Can you work these out from the model? Positions are in its coordinate system, mm. Give positions to 0.01 mm unless a question says otherwise; leave off trailing zeros. Loops run counter-clockwise (first coordinate to the right, second up) from the corner with the lowest first, then second, coordinate; pieces in that order, holes last. Notation, with made-up numbers: (-28, 9.25) -> (28, 9.25) arc R23 ccw to (28, 43.25) -> close; hole circle Ø8 at (32.25, 65.25). An arc over 180 degrees is marked (long way). Return JSON: item names as keys, results as strings. Group by question number.
Q1. Suppose I cut it at A-A, the plane y = 1.5. Count the separate pieces of the cut face and the enclosed holes in it, and give its area (3 significant figures).
Q2. Will these pins go through, and if not, where does the flat tip stop? pin 1 (5 mm diameter, centred on y = 42, z = 17.5, fed in from +X); pin 2 (2 mm diameter, centred on x = -9, z = 16, fed in from +Y); pin 3 (1.5 mm diameter, centred on y = 15.5, z = 18, fed in from +X).
Q3. Suppose I cut it at B-B, the plane x = 0. Please give me the cut outline in (y, z), and give its area (3 significant figures).
Q4. Suppose I cut it at D-D, the plane x = -24. Please give me the cut outline in (y, z).
Q5. I need wall thicknesses on line 1 along Y through (x, z) = (25, 14); line 2 along X through (y, z) = (27, -2.5); line 3 along Z through (x, y) = (5.5, 51). Which ranges of each line are inside material? Lowest first, please. Write a range as [from, to].
Q6. Suppose I cut it at C-C, the plane z = 18.5. Please give me the cut outline in (x, y), and give its area (3 significant figures).
Q7. Thinking about a two-plate mould opening in X: for faces 1 (the flat face through (-14.546, 28.594, 22.255)), 2 (the flat face through (1, 0, 1)), 3 (the flat face through (14.66, 28.59, 22.32)), 4 (the flat face through (0, 58, 24)), which applies, pulls with the +X half, pulls with the -X half, needs draft (parallel to the pull), parting line crosses it, or undercut?
```python
from build123d import *

# Parameters (mm, degrees)
SKETCH1_R           = 31
BOSS_EXTRUDE1_DEPTH = 50
SKETCH2_R           = 12.5
CUT_EXTRUDE1_DEPTH  = 50
CUT_EXTRUDE2_DEPTH  = 50
SKETCH4_R           = 4
SKETCH4_R_2         = 2.5
CUT_EXTRUDE3_DEPTH  = 67.498120274
SKETCH6_R           = 31
BOSS_EXTRUDE2_DEPTH = 3
BOSS_EXTRUDE3_DEPTH = 8


with BuildPart() as part:
    # Sketch1 → Boss-Extrude1 (new body)
    with BuildSketch(Plane(origin=(0, 0, 0), x_dir=(1, 0, 0), z_dir=(0, 1, 0))):
        with Locations(Location((0, 0, 0), (0, 0, 270))):
            Circle(SKETCH1_R)
    extrude(amount=BOSS_EXTRUDE1_DEPTH)

    # Sketch2 → Cut-Extrude1 (cut)
    with BuildSketch(Plane(origin=(0, 50, 0), x_dir=(1, 0, 0), z_dir=(0, 1, 0))):
        with Locations(Location((0, 15.5, 0), (0, 0, 270))):
            Circle(SKETCH2_R)
        with Locations(Location((13.423393759, -7.75, 0), (0, 0, 270))):
            Circle(SKETCH2_R)
        with Locations(Location((-13.423393759, -7.75, 0), (0, 0, 270))):
            Circle(SKETCH2_R)
    extrude(amount=-CUT_EXTRUDE1_DEPTH, mode=Mode.SUBTRACT)

    # Sketch3 → Cut-Extrude2 (cut)
    with BuildSketch(Plane(origin=(0, 50, 0), x_dir=(1, 0, 0), z_dir=(0, 1, 0))):
        with BuildLine():
            ThreePointArc((-12, 19), (0, 28), (12, 19))
            Line((12, 19), (12, 28.583211856))
            ThreePointArc((12, 28.583211856), (0, 31), (-12, 28.583211856))
            Line((-12, 28.583211856), (-12, 19))
        make_face()
        with BuildLine():
            ThreePointArc((18.753787589, -24.683910773), (26.846787517, -15.5), (30.753787589, -3.899301083))
            Line((30.753787589, -3.899301083), (22.454482672, 0.892304845))
            ThreePointArc((22.454482672, 0.892304845), (24.248711306, -14), (10.454482672, -19.892304845))
            Line((10.454482672, -19.892304845), (18.753787589, -24.683910773))
        make_face()
        with BuildLine():
            Line((-22.454482672, 0.892304845), (-30.753787589, -3.899301083))
            ThreePointArc((-30.753787589, -3.899301083), (-26.846787517, -15.5), (-18.753787589, -24.683910773))
            Line((-18.753787589, -24.683910773), (-10.454482672, -19.892304845))
            ThreePointArc((-10.454482672, -19.892304845), (-24.248711306, -14), (-22.454482672, 0.892304845))
        make_face()
    extrude(amount=-CUT_EXTRUDE2_DEPTH, mode=Mode.SUBTRACT)

    # Sketch4 → Cut-Extrude3 (cut, through all)
    with BuildSketch(Plane(origin=(0, 50, 0), x_dir=(1, 0, 0), z_dir=(0, 1, 0))):
        Circle(SKETCH4_R)
        with Locations((-10.392304845, 6)):
            Circle(SKETCH4_R_2)
        with Locations((10.392304845, 6)):
            Circle(SKETCH4_R_2)
        with Locations((0, -12)):
            Circle(SKETCH4_R_2)
    extrude(amount=-CUT_EXTRUDE3_DEPTH, mode=Mode.SUBTRACT)


with BuildPart() as cut_extrude3_piece_1:
    # of the separate pieces the step leaves, piece 1, a body of its own (cut_extrude3_pieces)
    add(part.part.solids().sort_by_distance((-12.538976962, 0, -4.718673022))[0])



with BuildPart() as cut_extrude3_piece_2:
    # of the separate pieces the step leaves, piece 2, a body of its own (cut_extrude3_pieces)
    add(part.part.solids().sort_by_distance((-18.753787589, 0, 24.683910773))[0])


with BuildPart() as cut_extrude3_piece_3:
    # of the separate pieces the step leaves, piece 3, a body of its own (cut_extrude3_pieces)
    add(part.part.solids().sort_by_distance((12.538976962, 0, -4.718673022))[0])


with BuildPart() as cut_extrude3_piece_4:
    # of the separate pieces the step leaves, piece 4, a body of its own (cut_extrude3_pieces)
    add(part.part.solids().sort_by_distance((3.976230514, 0, -0.43542037))[0])


with BuildPart() as cut_extrude3_piece_5:
    # of the separate pieces the step leaves, piece 5, a body of its own (cut_extrude3_pieces)
    add(part.part.solids().sort_by_distance((-3.976230514, 0, -0.43542037))[0])


with BuildPart() as cut_extrude3_piece_6:
    # of the separate pieces the step leaves, piece 6, a body of its own (cut_extrude3_pieces)
    add(part.part.solids().sort_by_distance((-1.083982046, 0, 9.747227725))[0])


with BuildPart() as cut_extrude3_piece_1_1:
    add(cut_extrude3_piece_1.part)

    add(cut_extrude3_piece_2.part)  # Boss-Extrude2 merges Cut-Extrude3 piece 2

    add(cut_extrude3_piece_3.part)  # Boss-Extrude2 merges Cut-Extrude3 piece 3

    add(cut_extrude3_piece_4.part)  # Boss-Extrude2 merges Cut-Extrude3 piece 4

    add(cut_extrude3_piece_5.part)  # Boss-Extrude2 merges Cut-Extrude3 piece 5

    add(cut_extrude3_piece_6.part)  # Boss-Extrude2 merges Cut-Extrude3 piece 6
    # Sketch6 → Boss-Extrude2 (add)
    with BuildSketch(Plane.XZ):
        with Locations(Location((0, 0, 0), (0, 0, 127.226027599))):
            Circle(SKETCH6_R)
    extrude(amount=BOSS_EXTRUDE2_DEPTH)

    # Sketch7 → Boss-Extrude3 (add)
    with BuildSketch(Plane(origin=(0, 50, 0), x_dir=(1, 0, 0), z_dir=(0, 1, 0))):
        with BuildLine():
            Line((-10.454482672, -19.892304845), (-18.753787589, -24.683910773))
            ThreePointArc((-18.753787589, -24.683910773), (0, -31), (18.753787589, -24.683910773))
            Line((18.753787589, -24.683910773), (10.454482672, -19.892304845))
            ThreePointArc((10.454482672, -19.892304845), (5.574105702, -17.478241208), (2.182997772, -13.218409097))
            ThreePointArc((2.182997772, -13.218409097), (0, -14.5), (-2.182997772, -13.218409097))
            ThreePointArc((-2.182997772, -13.218409097), (-5.574105702, -17.478241208), (-10.454482672, -19.892304845))
        make_face()
        with BuildLine():
            Line((22.454482672, 0.892304845), (30.753787589, -3.899301083))
            ThreePointArc((30.753787589, -3.899301083), (26.846787517, 15.5), (12, 28.583211856))
            Line((12, 28.583211856), (12, 19))
            ThreePointArc((12, 19), (12.349548049, 13.566437746), (10.35597919, 8.499736075))
            ThreePointArc((10.35597919, 8.499736075), (12.557368355, 7.25), (12.538976962, 4.718673022))
            ThreePointArc((12.538976962, 4.718673022), (17.923653751, 3.911803463), (22.454482672, 0.892304845))
        make_face()
        with BuildLine():
            Line((-12, 19), (-12, 28.583211856))
            ThreePointArc((-12, 28.583211856), (-26.846787517, 15.5), (-30.753787589, -3.899301083))
            Line((-30.753787589, -3.899301083), (-22.454482672, 0.892304845))
            ThreePointArc((-22.454482672, 0.892304845), (-17.923653751, 3.911803463), (-12.538976962, 4.718673022))
            ThreePointArc((-12.538976962, 4.718673022), (-12.557368355, 7.25), (-10.35597919, 8.499736075))
            ThreePointArc((-10.35597919, 8.499736075), (-12.349548049, 13.566437746), (-12, 19))
        make_face()
        with BuildLine():
            ThreePointArc((1.083982046, -9.747227725), (0, -9.5), (-1.083982046, -9.747227725))
            ThreePointArc((-1.083982046, -9.747227725), (-0.97000408, -6.671535571), (-1.611030155, -3.661226821))
            ThreePointArc((-1.611030155, -3.661226821), (0, -4), (1.611030155, -3.661226821))
            ThreePointArc((1.611030155, -3.661226821), (0.97000408, -6.671535571), (1.083982046, -9.747227725))
        make_face()
        with BuildLine():
            ThreePointArc((7.899355803, 5.812369851), (8.227241336, 4.75), (8.983337849, 3.934857873))
            ThreePointArc((8.983337849, 3.934857873), (6.262721327, 2.49571961), (3.976230514, 0.43542037))
            ThreePointArc((3.976230514, 0.43542037), (3.464101615, 2), (2.365200359, 3.225806452))
            ThreePointArc((2.365200359, 3.225806452), (5.292717247, 4.175815961), (7.899355803, 5.812369851))
        make_face()
        with BuildLine():
            ThreePointArc((-8.983337849, 3.934857873), (-8.227241336, 4.75), (-7.899355803, 5.812369851))
            ThreePointArc((-7.899355803, 5.812369851), (-5.292717247, 4.175815961), (-2.365200359, 3.225806452))
            ThreePointArc((-2.365200359, 3.225806452), (-3.464101615, 2), (-3.976230514, 0.43542037))
            ThreePointArc((-3.976230514, 0.43542037), (-6.262721327, 2.49571961), (-8.983337849, 3.934857873))
        make_face()
    extrude(amount=BOSS_EXTRUDE3_DEPTH)


solid = cut_extrude3_piece_1_1.part
```
Ans:
{
 "1": {"separate pieces": "6", "enclosed holes": "0", "area": "1,130 mm^2"},
 "2": {"pin 1": "stops at x = 10.64", "pin 2": "stops at y = 0", "pin 3": "stops at x = 7.49"},
 "3": {"outline": "(-3, -31) -> (0, -31) -> (0, 4) -> (58, 4) -> (58, 9.5) -> (0, 9.5) -> (0, 14.5) -> (58, 14.5) -> (58, 31) -> (-3, 31) -> close", "area": "1,460 mm^2"},
 "4": {"outline": "(-3, -19.62) -> (58, -19.62) -> (58, 0) -> (0, 0) -> (0, 19.62) -> (-3, 19.62) -> close"},
 "5": {"line 1": "y = [-3, 0]", "line 2": "x = [-30.9, -20.58], [-6.27, -3.12], [3.12, 6.27], [20.58, 30.9]", "line 3": "z = [-4.28, -1.92], [17.42, 30.51]"},
 "6": {"outline": "(-24.87, -3) -> (24.87, -3) -> (24.87, 0) -> (7.04, 0) -> (7.04, 58) -> (-7.04, 58) -> (-7.04, 0) -> (-24.87, 0) -> close", "area": "966 mm^2"},
 "7": {"face 1": "pulls with the -X half", "face 2": "undercut", "face 3": "pulls with the +X half", "face 4": "needs draft"}
}
